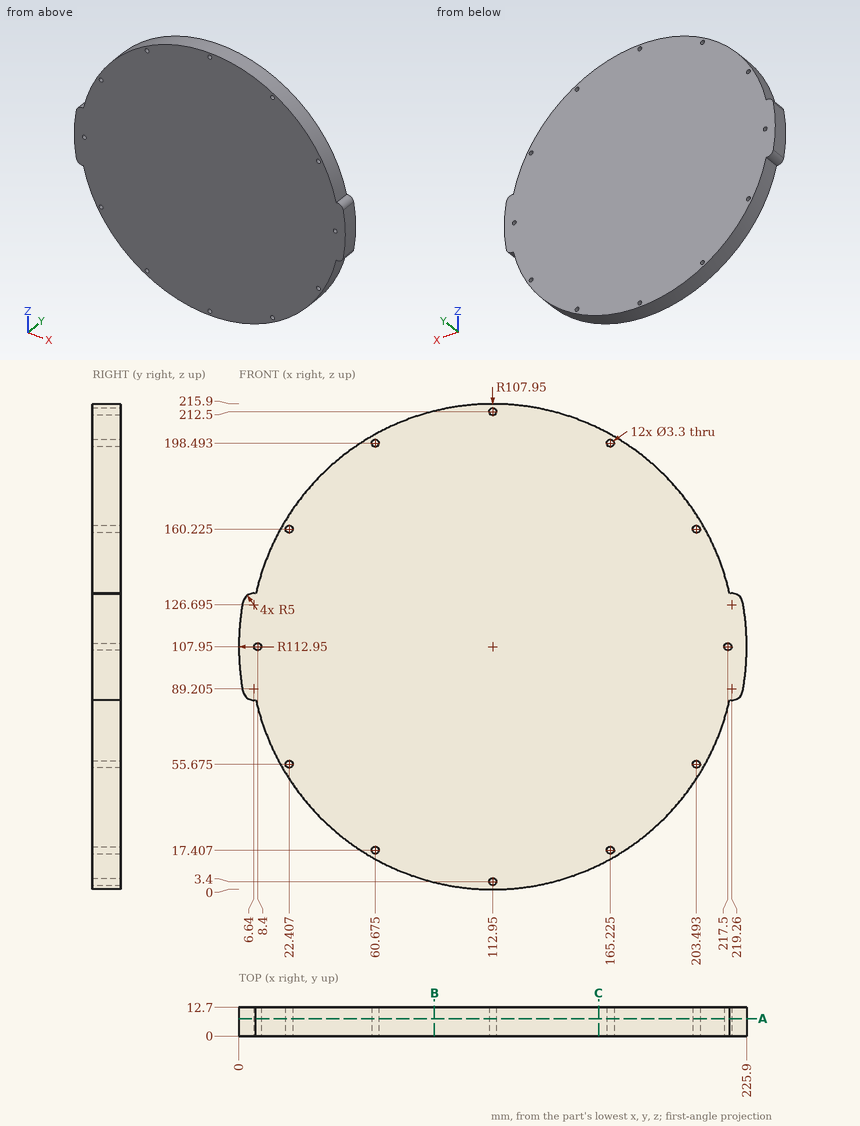
Print and shaded views of the part. All mm, measured from the part's lowest x, y and z. Give positions to 0.01 mm unless a question says otherwise; leave off trailing zeros. Write each loop counter-clockwise with the first axis right and the second up, starting at its lowest first coordinate (ties: lowest second). Pieces come first, ordered by that corner, then holes. Notation, with made-up numbers: (-19, 63) -> (40, 63) arc R15 cw to (40, 80) -> close; hole circle Ø1 at (35.25, 55). An arc over 180 degrees is marked (long way). Write item = value, one per line.
(1) Slice it at C-C, the plane x = 160. Give the cut face in (y, z), then the cut area to 3 significant figures.
Determined:
outline = (0, 10.79) -> (12.7, 10.79) -> (12.7, 205.11) -> (0, 205.11) -> close
area = 2,470 mm2
(2) Slice it at A-A, the plane y = 7.75. Give the number of separate pieces and of enclosed holes in the cut face, then the cut area to 3 significant figures.
Determined:
separate_pieces = 1
enclosed_holes = 12
area = 37,000 mm2
(3) Slice it at B-B, the plane x = 87. Give the cut face in (y, z) (1 decimal).
Determined:
outline = (0, 3.2) -> (12.7, 3.2) -> (12.7, 212.7) -> (0, 212.7) -> close
(4) Probe line 1 along X through (y, z) = (5, 107.95); line 2 along X through (y, z) = (10.5, 106); line 3 along Z through (x, y) = (31, 9) (1 decimal). List the from-to ranges inside material, lowest first.
Determined:
line_1 = 0 to 6.75, 10.05 to 215.85, 219.15 to 225.9
line_2 = 0.02 to 225.88
line_3 = 37.7 to 178.2
(5) Flat gauge pins, fed straight in: P1, Ø1.5, axis at x = 179.5, y = 10, coming from the +Z side; P2, Ø2.5, axis at x = 22.41, z = 160.22, coming from the +Y side; P3, Ø6, axis at y = 4, z = 139.5, coming from the +X side; P4, Ø1, axis at x = 186, y = 6, coming from the +Z side (1 decimal). Where does each tip first touch, or does it go through?
Determined:
P1 = 193.53
P2 = through
P3 = 217.06
P4 = 187.9
